```python
from build123d import *

# Parameters (mm, degrees)
SKETCH1_W           = 6
SKETCH1_H           = 12
BOSS_EXTRUDE1_DEPTH = 6
SKETCH3_R           = 0.5
CUT_EXTRUDE1_DEPTH  = 7


with BuildPart() as part:
    # Sketch1 → Boss-Extrude1 (new body)
    with BuildSketch(Plane.XY):
        Polygon((-124, 38), (-124, 32), (-124, 20), (-124, -20), (-124, -32), (-124, -38), (-71, -38), (-71, -32), (-59, -32), (-59, -38), (-6, -38), (-6, -32), (6, -32), (6, -38), (59, -38), (59, -32), (71, -32), (71, -38), (124, -38), (124, -32), (124, -20), (124, 20), (124, 32), (124, 38), align=None)
        with Locations((-107, -20)):
            Rectangle(SKETCH1_W, SKETCH1_H, mode=Mode.SUBTRACT)
        with Locations((-107, 22)):
            Rectangle(SKETCH1_W, SKETCH1_H, mode=Mode.SUBTRACT)
        with Locations((-127, -26)):
            Rectangle(SKETCH1_W, SKETCH1_H)
        with Locations((-127, 26)):
            Rectangle(SKETCH1_W, SKETCH1_H)
        with Locations((127, 26)):
            Rectangle(SKETCH1_W, SKETCH1_H)
        with Locations((127, -26)):
            Rectangle(SKETCH1_W, SKETCH1_H)
    extrude(amount=-BOSS_EXTRUDE1_DEPTH)

    # Sketch3 → Cut-Extrude1 (cut, through all)
    with BuildSketch(Plane.XY):
        with Locations((-107, -29)):
            Circle(SKETCH3_R)
    extrude(amount=-CUT_EXTRUDE1_DEPTH, mode=Mode.SUBTRACT)


solid = part.part
```
Input: part model. Units: mm. Frame: model coordinates. A direction names the side the tool comes from. Round coordinates to 2 decimals unless told otherwise and drop trailing zeros. Loops run counter-clockwise (first coordinate to the right, second up) from the corner with the lowest first, then second, coordinate; pieces in that order, holes last. Notation, with made-up numbers: (-3.5, 12.25) - (1.5, 12.25) arc R15 cw to (1.5, 41.25) - close; hole circle Ø6 at (66.5, 48.25). An arc over 180 degrees is marked (long way). One line per item, written item: value. Start each with the question number.
(1) Draft query along X for faces 5 (the flat face through (124, 0, -3)), 6 (the flat face through (-127, -32, -3)), 7 (the flat face through (-130, -26, -3)), 8 (the flat face through (-71, -35, -3)). Return one class per face: +X half, -X half, draft (parallel to the pull), parting line (faces both ways), or undercut.
(2) Access query for faces 1 (the flat face through (-127, 20, -3)), 2 (the flat face through (127, 20, -3)), 3 (the flat face through (-107, 28, -3)), 4 (the flat face through (59, -35, -3)). Directions: +Z, -Z, +X, -X, +Y, -Y. A direction counts if a zero-diameter tool reaches every point of the face in a straight line with its end or side. Return the directions, or none.
(3) Ray query, line 1 (Y direction, x = -107, z = -4.35); line 2 (Y direction, x = -105.5, z = -3.35); line 3 (X direction, y = -18, z = -4.95). Return the intervals inside material, ascending. Write a range as [from, to].
(4) Section B-B, the plane z = -1.4. Count the separate pieces of the cut face and the enclosed holes in it, plus the area to 3 significant figures.
(5) Contact query for flat-ended pins moving along their axis: P1, Ø3, axis at y = -34.5, z = -3.5, coming from the -X side; P2, Ø1.8, axis at x = 127.5, z = -3, coming from the -Y side; P3, Ø3, axis at y = -34, z = -3.5, coming from the +X side. Output: stop coordinate, or through.
(6) Section D-D, the plane y = 3. Return loops of the section in (x, z).
(7) Section A-A, the plane y = -22.5. Return loops of the section in (x, z), plus the area to 3 significant figures.
(8) Section C-C, the plane x = -67. Return loops of the section in (y, z), plus the area to 3 significant figures.
Results below:
1. face 5: +X half
1. face 6: draft
1. face 7: -X half
1. face 8: undercut
2. face 1: +Z, -Z, -X
2. face 2: +Z, -Z, +X
2. face 3: +Z, -Z
2. face 4: +Z, -Z, -Y
3. line 1: [-38, -29.5], [-28.5, -26], [-14, 16], [28, 38]
3. line 2: [-38, -26], [-14, 16], [28, 38]
3. line 3: [-124, -110], [-104, 124]
4. separate pieces: 1
4. enclosed holes: 3
4. area: 18,800 mm^2
5. P1: x = -124
5. P2: y = -32
5. P3: x = 124
6. outline: (-124, -6) - (124, -6) - (124, 0) - (-124, 0) - close
7. outline: (-130, -6) - (-110, -6) - (-110, 0) - (-130, 0) - close; (-104, -6) - (130, -6) - (130, 0) - (-104, 0) - close
7. area: 1,520 mm^2
8. outline: (-32, -6) - (38, -6) - (38, 0) - (-32, 0) - close
8. area: 420 mm^2
